from build123d import *

# Parameters (mm, degrees)
F0_W     = 6.9
F0_H     = 1
F0_W_2   = 1
F0_H_2   = 7.5
F0_W_3   = 2.5
F0_H_3   = 2.5
F3_DEPTH = 2.5


with BuildPart() as f1:
    # F0 (on Front) → F1 (revolve)
    with BuildSketch(Plane.XZ):
        Polygon((1, -1), (0, 0), (-2.5, 0), (-2.5, -1), align=None)
        with Locations((-5.95, -0.5)):
            Rectangle(F0_W, F0_H)
    revolve(axis=Axis((-4.7, 0, 0), (-1, 0, 0)))

    # F0 (on Front) → F2 (revolve)
    with BuildSketch(Plane.XZ):
        with Locations((0.5, 6.25)):
            Rectangle(F0_W_2, F0_H_2)
        Polygon((0, 2.5), (0, 0), (1, -1), (1, 2.5), align=None)
    revolve(axis=Axis((0, 0, 5), (0, 0, 1)))

    # F0 (on Front) → F3 (join, symmetric)
    with BuildSketch(Plane.XZ):
        Polygon((1, 2.5), (1, -1), (-2.5, -1), (-2.5, -2.5), (2.5, -2.5), (2.5, 2.5), align=None)
        with Locations((-1.25, 1.25)):
            Rectangle(F0_W_3, F0_H_3)
        Polygon((0, 2.5), (0, 0), (1, -1), (1, 2.5), align=None)
        Polygon((1, -1), (0, 0), (-2.5, 0), (-2.5, -1), align=None)
    extrude(amount=F3_DEPTH, both=True)


solid = f1.part
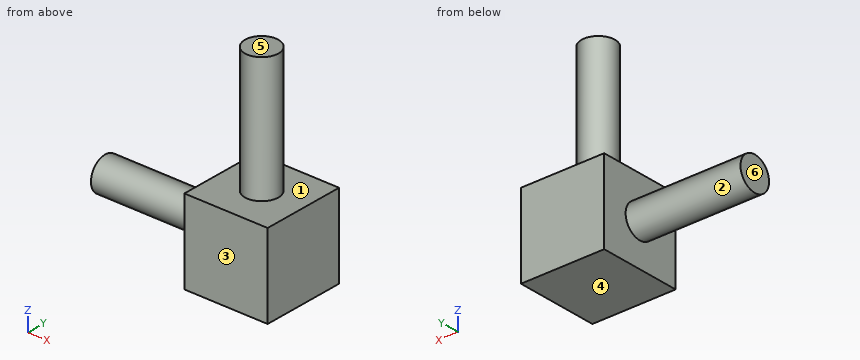
Could you check a few things on this model? Use its own coordinates, in mm. Face numbers are marked on the shaded views. A direction names the side the tool comes from. Coordinates: 2 decimals unless noted, no trailing zeros. Write each loop counter-clockwise with the first axis right and the second up, starting at its lowest first coordinate (ties: lowest second). Pieces come first, ordered by that corner, then holes. Notation, with made-up numbers: (10, 46.5) - (34, 46.5) arc R30 ccw to (34, 75.5) - close; hole circle Ø8 at (31, -38). An arc over 180 degrees is marked (long way). Write item = value, one per line.
1) Suppose I cut it at A-A on x = 0. Please give me the cut outline in (y, z).
Result set:
outline = (-2.5, -2.5) - (2.5, -2.5) - (2.5, 2.5) - (1, 2.5) - (1, 10) - (-1, 10) - (-1, 2.5) - (-2.5, 2.5) - close
2) Suppose I cut it at D-D on y = 0.7. Please give me the cut outline in (x, z).
Result set:
outline = (-9.4, -0.71) - (-2.5, -0.71) - (-2.5, -2.5) - (2.5, -2.5) - (2.5, 2.5) - (0.71, 2.5) - (0.71, 10) - (-0.71, 10) - (-0.71, 2.5) - (-2.5, 2.5) - (-2.5, 0.71) - (-9.4, 0.71) - close
3) Please list where these lines run through material, in increasing order: line 1 (Z direction, x = 1, y = 0.7); line 2 (Z direction, x = -5.25, y = -0.6); line 3 (X direction, y = 0.75, z = 5). Write a range as [from, to].
Result set:
line_1 = [-2.5, 2.5]
line_2 = [-0.8, 0.8]
line_3 = [-0.66, 0.66]
4) Suppose I cut it at C-C on y = 0. Please give me the cut outline in (x, z), plus the area to 3 significant figures.
Result set:
outline = (-9.4, -1) - (-2.5, -1) - (-2.5, -2.5) - (2.5, -2.5) - (2.5, 2.5) - (1, 2.5) - (1, 10) - (-1, 10) - (-1, 2.5) - (-2.5, 2.5) - (-2.5, 1) - (-9.4, 1) - close
area = 53.8 mm2
5) We'd pull the mould along Z, two halves only. Please class the marked faces 4, 5 and 6: +Z half, -Z half, draft (parallel to the pull), parting line (faces both ways), or undercut.
Result set:
face_4 = -Z half
face_5 = +Z half
face_6 = draft
6) For the marked faces 1, 2 and 3, which set-ups out of +Z, -Z, +X, -X, +Y, -Y let a thin tool reach every point of the face, with its end or its side?
Result set:
face_1 = +Z
face_2 = -X
face_3 = +Z, -Z, +X, -X, -Y
7) Will these pins go through, and if not, where does the flat tip stop? pin 1 Ø3 at (x, y) = (-0.5, 1) entering from +Z; pin 2 Ø1 at (x, y) = (-4, -2) entering from +Z; pin 3 Ø2 at (x, z) = (-4.5, -1) entering from +Y.
Result set:
pin_1 = 10
pin_2 = through
pin_3 = 1
8) Suppose I cut it at B-B on z = 0. Please give me the cut outline in (x, y).
Result set:
outline = (-9.4, -1) - (-2.5, -1) - (-2.5, -2.5) - (2.5, -2.5) - (2.5, 2.5) - (-2.5, 2.5) - (-2.5, 1) - (-9.4, 1) - close
